from build123d import *

# Parameters (mm, degrees)
SKETCH2_W            = 220
SKETCH2_H            = 90
BOSS_EXTRUDE1_DEPTH  = 4.5
SKETCH3_W            = 20.25
SKETCH3_H            = 4.65
CUT_EXTRUDE1_DEPTH   = 119.933805119
SKETCH4_W            = 31.802775074
SKETCH4_H            = 10
INPUT_LINK_CUT_DEPTH = 119.933805119


with BuildPart() as part:
    # Sketch2 → Boss-Extrude1 (new body)
    with BuildSketch(Plane(origin=(0, 0, 0), x_dir=(1, 0, 0), z_dir=(0, 1, 0))):
        Rectangle(SKETCH2_W, SKETCH2_H)
    extrude(amount=BOSS_EXTRUDE1_DEPTH)

    # Sketch3 → Cut-Extrude1 (cut, through all)
    with BuildSketch(Plane.XZ):
        with Locations((40, -15)):
            Rectangle(SKETCH3_W, SKETCH3_H)
        with Locations((0, -15)):
            Rectangle(SKETCH3_W, SKETCH3_H)
        with Locations((80, -15)):
            Rectangle(SKETCH3_W, SKETCH3_H)
        with Locations((-80, -15)):
            Rectangle(SKETCH3_W, SKETCH3_H)
        with Locations((-40, -15)):
            Rectangle(SKETCH3_W, SKETCH3_H)
    extrude(amount=-CUT_EXTRUDE1_DEPTH, mode=Mode.SUBTRACT)

    # Sketch4 → Input link cut (cut, through all)
    with BuildSketch(Plane.XZ):
        with Locations((40, 2)):
            Rectangle(SKETCH4_W, SKETCH4_H)
    extrude(amount=-INPUT_LINK_CUT_DEPTH, mode=Mode.SUBTRACT)


solid = part.part
The model under review builds one solid part; all positions refer to its coordinate system, in mm. A direction names the side the tool comes from. Round coordinates to 2 decimals unless told otherwise and drop trailing zeros. Loops run counter-clockwise (first coordinate to the right, second up) from the corner with the lowest first, then second, coordinate; pieces in that order, holes last. Notation, with made-up numbers: (80.5, -19.5) -> (117.5, -19.5) arc R29 ccw to (117.5, 5.5) -> close; hole circle Ø8 at (66, 42.25). An arc over 180 degrees is marked (long way). Write item = value, one per line. Start each with the question number.
Item 1: For faces 3 (the flat face through (-2, 4.5, -1)), 4 (the flat face through (50.125, 2, -15)), list the 3-axis set-ups (+Z, -Z, +X, -X, +Y, -Y) from which the entire face can be reached by the end or side of a thin tool; tool diameter is ignored.
Item 2: Mouldability with a two-part tool opening along Z and no side actions: class faces 1 (the flat face through (90.125, 2, -15)), 2 (the flat face through (-2, 0, -1)) as released by +Z, released by -Z, zero draft, split by the parting line, or undercut.
Item 3: Take a section at A-A on x = -43. Give the boundary of the cut face in (y, z) (3 decimals), plus the area to 3 significant figures.
Item 4: Take a section at C-C on y = 2.4. Give the boundary of the cut face in (x, z) (3 decimals).
Item 5: To check wall thickness, follow L1, parallel to X at y = 3.4, z = -13 (3 decimals); L2, parallel to Z at x = 39.5, y = 1.15 (3 decimals); L3, parallel to Z at x = -75, y = 4 (3 decimals). State the ranges of each line that lie inside material, in increasing order.
Item 6: Take a section at B-B on x = 42. Give the boundary of the cut face in (y, z) (3 decimals), plus the area to 3 significant figures.
Result:
q1.face_3 = +Z, -Z, +X, -X, +Y
q1.face_4 = +Y, -Y
q2.face_1 = undercut
q2.face_2 = zero draft
q3.outline = (0, -45) -> (4.5, -45) -> (4.5, -17.325) -> (0, -17.325) -> close; (0, -12.675) -> (4.5, -12.675) -> (4.5, 45) -> (0, 45) -> close
q3.area = 384 mm²
q4.outline = (-110, -45) -> (110, -45) -> (110, 45) -> (-110, 45) -> close; hole (-90.125, -17.325) -> (-69.875, -17.325) -> (-69.875, -12.675) -> (-90.125, -12.675) -> close; hole (-50.125, -17.325) -> (-29.875, -17.325) -> (-29.875, -12.675) -> (-50.125, -12.675) -> close; hole (-10.125, -17.325) -> (10.125, -17.325) -> (10.125, -12.675) -> (-10.125, -12.675) -> close; hole (24.099, -3) -> (55.901, -3) -> (55.901, 7) -> (24.099, 7) -> close; hole (29.875, -17.325) -> (50.125, -17.325) -> (50.125, -12.675) -> (29.875, -12.675) -> close; hole (69.875, -17.325) -> (90.125, -17.325) -> (90.125, -12.675) -> (69.875, -12.675) -> close
q5.L1 = -110 to -90.125, -69.875 to -50.125, -29.875 to -10.125, 10.125 to 29.875, 50.125 to 69.875, 90.125 to 110
q5.L2 = -45 to -17.325, -12.675 to -3, 7 to 45
q5.L3 = -45 to -17.325, -12.675 to 45
q6.outline = (0, -45) -> (4.5, -45) -> (4.5, -17.325) -> (0, -17.325) -> close; (0, -12.675) -> (4.5, -12.675) -> (4.5, -3) -> (0, -3) -> close; (0, 7) -> (4.5, 7) -> (4.5, 45) -> (0, 45) -> close
q6.area = 339 mm²
